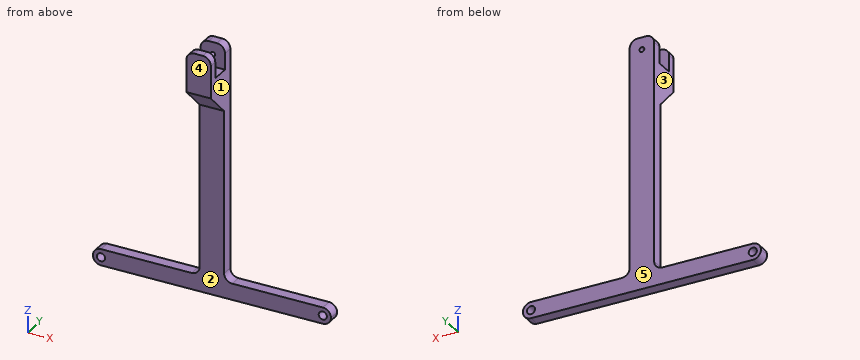
```python
from build123d import *

# Parameters (mm, degrees)
SALIENTE_EXTRUIR1_DEPTH = 7.5
CROQUIS4_R              = 1.5
CORTAR_EXTRUIR2_DEPTH   = 6
CROQUIS5_W              = 146
CROQUIS5_H              = 10
CROQUIS5_R              = 2.5
SALIENTE_EXTRUIR2_DEPTH = 7
REDONDEO2_R             = 5


with BuildPart() as part:
    # Croquis1 → Saliente-Extruir1 (new, symmetric)
    with BuildSketch(Plane(origin=(0, 0, 0), x_dir=(0, 0, -1), z_dir=(1, 0, 0))):
        Polygon((0, 0), (0, 11), (-15, 11), (-15, 17), (140, 17), (140, 10), (25, 10), (10, -5), (-15, -5), (-15, 0), align=None)
    extrude(amount=SALIENTE_EXTRUIR1_DEPTH, both=True)

    # Croquis4 → Cortar-Extruir2 (cut)
    with BuildSketch(Plane(origin=(0, 17, 0), x_dir=(1, 0, 0), z_dir=(0, 1, 0))):
        with Locations(Location((0, -7.5, 0), (0, 0, 270))):
            Circle(CROQUIS4_R)
    extrude(amount=-CORTAR_EXTRUIR2_DEPTH, mode=Mode.SUBTRACT)

    # Croquis5 → Saliente-Extruir2 (add)
    with BuildSketch(Plane(origin=(0, 17, 0), x_dir=(1, 0, 0), z_dir=(0, 1, 0))):
        with Locations((0, 135)):
            Rectangle(CROQUIS5_W, CROQUIS5_H)
        with Locations(Location((-68, 135, 0), (0, 0, 270))):
            Circle(CROQUIS5_R, mode=Mode.SUBTRACT)
        with Locations(Location((68, 135, 0), (0, 0, 270))):
            Circle(CROQUIS5_R, mode=Mode.SUBTRACT)
    extrude(amount=-SALIENTE_EXTRUIR2_DEPTH)

    # Redondeo2
    redondeo2_edges = [part.edges().sort_by_distance(p)[0] for p in [
        (-7.5, 13.5, -130),
        (-73, 13.5, -140),
        (-73, 13.5, -130),
        (7.5, 13.5, -130),
        (7.5, -2.5, 15),
        (-7.5, -2.5, 15),
        (-7.5, 14, 15),
        (7.5, 14, 15),
        (73, 13.5, -140),
        (73, 13.5, -130),
    ]]
    fillet(redondeo2_edges, radius=REDONDEO2_R - 0.0001)  # a hair under: the kernel refuses the full size


solid = part.part
```
Geometry check sheet. Reference: the model listing, model coordinates, mm. Face numbers are marked on the shaded views. A direction names the side the tool comes from. Round coordinates to 2 decimals unless told otherwise and drop trailing zeros. Order: outer loops, then holes, each group sorted by start corner. A loop starts at its lowest first (then second) coordinate and runs counter-clockwise, first axis right, second up. Notation, with made-up numbers: (79.25, 47.5) - (111.25, 47.5) arc R29 ccw to (111.25, 83.5) - close; hole circle Ø8 at (-14.75, -28.5). An arc over 180 degrees is marked (long way). Use a Markdown table: item, result. Add a question column.
1) Gauge pin test, flat ends, axial feed: P1, Ø7.5, axis at x = -45, y = 12.5, coming from the +Z side; P2, Ø12, axis at x = -2.5, y = 8, coming from the +Z side; P3, Ø6, axis at y = 10, z = -16.5, coming from the +X side; P4, Ø8, axis at x = -68, z = -135, coming from the -Y side. Record the tip position at first contact, or that the pin passes through.
2) Section check C-C (x = -58.5). Record the cut outline in (y, z), then the cut area to 3 significant figures.
3) Section check D-D (z = -105.5). Record the cut outline in (x, y).
4) Set-up check for the marked faces 1, 2, 3, 4 and 5: record each of +Z, -Z, +X, -X, +Y, -Y from which the full face is reachable in a straight line by a thin tool's end or side.
5) Section check A-A (y = 13.75). Count the separate pieces of the cut face and the enclosed holes in it, then the cut area to 3 significant figures.
6) Thickness scan on line 1 along X through (y, z) = (12.5, -135); line 2 along X through (y, z) = (12.95, 7.5); line 3 along Z through (x, y) = (-44.5, 11.25). Record the ranges inside material, lowest first.
7) Section check B-B (y = -2.5). Record the cut outline in (x, z).
Established:
| question | item | result |
|---|---|---|
| 1 | P1 | z = -130 |
| 1 | P2 | z = 15 |
| 1 | P3 | x = 7.5 |
| 1 | P4 | y = 10 |
| 2 | outline | (10, -140) - (17, -140) - (17, -130) - (10, -130) - close |
| 2 | area | 70.0 mm2 |
| 3 | outline | (-7.5, 10) - (7.5, 10) - (7.5, 17) - (-7.5, 17) - close |
| 4 | face 1 | +Z, +X, +Y, -Y |
| 4 | face 2 | -Z, +X, -X, -Y |
| 4 | face 3 | +Z, -X, +Y, -Y |
| 4 | face 4 | +Z, -Z, +X, -X, -Y |
| 4 | face 5 | +Z, -Z, +X, -X, +Y |
| 5 | separate pieces | 1 |
| 5 | enclosed holes | 3 |
| 5 | area | 3,570 mm2 |
| 6 | line 1 | -73 to -70.5, -65.5 to 65.5, 70.5 to 73 |
| 6 | line 2 | -7.5 to -1.5, 1.5 to 7.5 |
| 6 | line 3 | -140 to -130 |
| 7 | outline | (-7.5, -12.5) - (7.5, -12.5) - (7.5, 10) arc R5 ccw to (2.5, 15) - (-2.5, 15) arc R5 ccw to (-7.5, 10) - close |
